```python
from build123d import *

# Parameters (mm, degrees)
SKETCH1_R           = 0.5
BOSS_EXTRUDE1_DEPTH = 15.5
BOSS_EXTRUDE2_START = -4.75
SKETCH1_3_R         = 1.2
SKETCH1_3_R_2       = 0.5
BOSS_EXTRUDE2_DEPTH = 4.75
FILLET1_R           = 0.2
SKETCH2_R           = 0.85
BOSS_EXTRUDE3_DEPTH = 0.3
SKETCH4_W           = 0.445498432
SKETCH4_H           = 0.1
SKETCH5_W           = 0.773123016
SKETCH5_H           = 2.46
SKETCH5_2_W         = 0.773123016
SKETCH5_2_H         = 2.46


with BuildPart() as part:
    # Sketch1 → Boss-Extrude1 (new body)
    with BuildSketch(Plane.XY):
        Circle(SKETCH1_R)
    extrude(amount=BOSS_EXTRUDE1_DEPTH)

    # Sketch1_3 → Boss-Extrude2 (add)
    # profile 1 of 2: a face of its own
    with BuildSketch(Plane.XY.offset(BOSS_EXTRUDE2_START)):
        with Locations((0.031563249, 0)):
            Circle(SKETCH1_3_R)
        Circle(SKETCH1_3_R_2, mode=Mode.SUBTRACT)
    # profile 2 of 2: a face of its own
    with BuildSketch(Plane.XY.offset(BOSS_EXTRUDE2_START)):
        Circle(SKETCH1_3_R_2)
    extrude(amount=BOSS_EXTRUDE2_DEPTH)

    # Fillet1
    fillet1_edges = [part.edges().sort_by_distance(p)[0] for p in [
        (-1.168436751, 0, 0),
    ]]
    fillet(fillet1_edges, radius=FILLET1_R)

    # Sketch2 → Boss-Extrude3 (add)
    with BuildSketch(Plane.XY):
        Circle(SKETCH2_R)
    extrude(amount=BOSS_EXTRUDE3_DEPTH)

    # Sketch3 → Revolve2 (revolve)
    with BuildSketch(Plane(origin=(0, 0, 0), x_dir=(1, 0, 0), z_dir=(0, 1, 0)), mode=Mode.PRIVATE) as revolve2_sk:
        with BuildLine():
            Line((0, -15.5), (0, -16.0775))
            ThreePointArc((0, -16.0775), (0.247487373, -16.180012627), (0.35, -16.4275))
            Line((0.35, -16.4275), (0.5, -16.4275))
            ThreePointArc((0.5, -16.4275), (0.460977223, -16.233850833), (0.35, -16.070428579))
            Line((0.35, -16.070428579), (0.35, -15.970428579))
            Line((0.35, -15.970428579), (0.5, -15.970428579))
            Line((0.5, -15.970428579), (0.5, -15.770428579))
            Line((0.5, -15.770428579), (0.4, -15.770428579))
            ThreePointArc((0.4, -15.770428579), (0.430084247, -15.627849774), (0.5, -15.5))
            Line((0.5, -15.5), (0, -15.5))
        make_face()
    revolve(revolve2_sk.sketch.rotate(Axis((0, 0, 15.5), (0, 0, 1)), 180), axis=Axis((0, 0, 15.5), (0, 0, 1)))

    # Sketch4 → Revolve3 (revolve)
    with BuildSketch(Plane(origin=(0, 0, 0), x_dir=(1, 0, 0), z_dir=(0, 1, 0))):
        with Locations((-0.222202563, -16.29)):
            Rectangle(SKETCH4_W, SKETCH4_H)
    revolve(axis=Axis((0.000546653, 0, 16.34), (0, 0, -1)))

    # Sketch5 → Revolve4 (revolve)
    with BuildSketch(Plane(origin=(0, 0, 0), x_dir=(1, 0, 0), z_dir=(0, 1, 0))):
        with Locations((-0.686561508, -14.27)):
            Rectangle(SKETCH5_W, SKETCH5_H)
    revolve(axis=Axis((0, 0, 15.5), (0, 0, 1)))

    # Sketch5_2 → Cut-Revolve1 (revolve, cut)
    with BuildSketch(Plane(origin=(0, 0, 0), x_dir=(1, 0, 0), z_dir=(0, 1, 0))):
        with Locations((-0.686561508, -14.27)):
            Rectangle(SKETCH5_2_W, SKETCH5_2_H)
    revolve(axis=Axis((0, 0, 15.5), (0, 0, 1)), mode=Mode.SUBTRACT)


solid = part.part
```
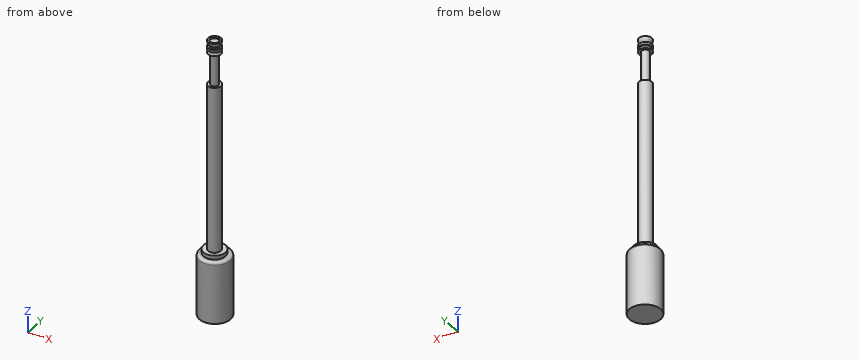
For this review, take the finished solid that the model builds, in its own axes (mm). Round coordinates to 2 decimals unless told otherwise and drop trailing zeros. Loops run counter-clockwise (first coordinate to the right, second up) from the corner with the lowest first, then second, coordinate; pieces in that order, holes last.
Q1. Insertion check: pin 1 Ø0.5 at (x, y) = (0, 0) entering from +Z. The pin has a flat end and moves straight along its axis. Give the tip position at first contact, or say it passes through.
Result sheet:
pin 1: stops at z = 16.34
Q2. Add section A-A on z = 7.25. Write out the cut boundary in (x, y), plus the area to 3 significant figures.
Result sheet:
outline: circle Ø1 at (0, 0)
area: 0.785 mm2
Q3. To check wall thickness, follow line 1 along Z through (x, y) = (0.2, 0.9); line 2 along X through (y, z) = (0.05, 11.25); line 3 along Y through (x, z) = (0.4, 6.75). State the ranges of each line that lie inside material, in increasing order.
Result sheet:
line 1: z = -4.75 to 0
line 2: x = -0.5 to 0.5
line 3: y = -0.3 to 0.3
